Read the model definition and answer for the solid it produces. Units are mm, in the model's axes. A direction names the side the tool comes from. Round coordinates to 2 decimals unless told otherwise and drop trailing zeros. Write each loop counter-clockwise with the first axis right and the second up, starting at its lowest first coordinate (ties: lowest second). Pieces come first, ordered by that corner, then holes. Notation, with made-up numbers: (89, -33.75) -> (120, -33.75) arc R20 cw to (120, -23.75) -> close; hole circle Ø8 at (88, 85). An arc over 180 degrees is marked (long way). Return JSON: item names as keys, results as strings. Group by question number.
(1) The mould has two halves that part along Y. Classify faces 1 (the flat face through (0, -3.175, -7)), 2 (the cylindrical face through (-0.01, -5.62, 6.54)), 3 (the flat face through (-5, 1, -11.112)): released by +Y, released by -Y, zero draft, split by the parting line, or undercut.
(2) A cutting plane is placed at C-C on y = 0. Give the vertices of the cut face in (x, z) (1 decimal).
(3) A cutting plane is placed at A-A on z = 8.75. Give the vertices of the cut face in (x, y), then the cut area to 3 significant figures.
(4) A cutting plane is placed at D-D on z = -4.5. Give the vertices of the cut face in (x, y) (3 decimals), then the cut area to 3 significant figures.
(5) For faces 4 (the flat face through (-3.175, 0, -7)), 5 (the flat face through (2, 6, 11.112)), 6 (the cylindrical face through (-4.87, -2.8, 6.54)), determine the directions among +Z, -Z, +X, -X, +Y, -Y from which every point of the face is accessible in a straight line to the end or side of a thin tool.
(6) Straight lines are drawn through the part: line 1 (Y direction, x = 0, z = -1.05); line 2 (X direction, y = 0.25, z = -6.75) (3 decimals); line 3 (Z direction, x = -4.5, y = 3). For each, find the intervals that lie inside material, in ascending order.
(7) Given pin 1 (1.5 mm diameter, centred on y = 5.5, z = 8, fed in from +X); pin 2 (0.9 mm diameter, centred on x = 3.5, y = -1, fed in from +Z); pin 3 (7 mm diameter, centred on x = 0, y = 0, fed in from -Z), each flat-ended and moving along its own axis, determine where each tip first touches the part or whether it passes through.
```python
from build123d import *

# Parameters (mm, degrees)
SKETCH4_W          = 22.225
SKETCH4_H          = 7.3421875
CUT_EXTRUDE1_DEPTH = 9.128125
CUT_EXTRUDE3_START = -4.7625
SKETCH7_R          = 4
CUT_EXTRUDE3_DEPTH = 4.7625
SKETCH9_W          = 6.35
SKETCH9_H          = 6.35
CUT_EXTRUDE5_DEPTH = 8.334375
FILLET1_R          = 0.3175


with BuildPart() as part:
    # Sketch4 → Revolve1 (revolve)
    with BuildSketch(Plane(origin=(0, 0, 0), x_dir=(0, 0, -1), z_dir=(1, 0, 0)), mode=Mode.PRIVATE) as revolve1_sk:
        with Locations((0, 3.67109375)):
            Rectangle(SKETCH4_W, SKETCH4_H)
    revolve(revolve1_sk.sketch.rotate(Axis((0, 0, 11.1125), (0, 0, -1)), 90), axis=Axis((0, 0, 11.1125), (0, 0, -1)))

    # Sketch5 → Cut-Extrude1 (cut)
    with BuildSketch(Plane.XY.offset(11.1125)):
        with BuildLine():
            Line((-5, 2.309401077), (-5, -2.309401077))
            ThreePointArc((-5, -2.309401077), (-4.866025404, -2.809401077), (-4.5, -3.175426481))
            Line((-4.5, -3.175426481), (-0.5, -5.484827557))
            ThreePointArc((-0.5, -5.484827557), (0, -5.618802154), (0.5, -5.484827557))
            Line((0.5, -5.484827557), (4.5, -3.175426481))
            ThreePointArc((4.5, -3.175426481), (4.866025404, -2.809401077), (5, -2.309401077))
            Line((5, -2.309401077), (5, 2.309401077))
            ThreePointArc((5, 2.309401077), (4.866025404, 2.809401077), (4.5, 3.175426481))
            Line((4.5, 3.175426481), (0.5, 5.484827557))
            ThreePointArc((0.5, 5.484827557), (0, 5.618802154), (-0.5, 5.484827557))
            Line((-0.5, 5.484827557), (-4.5, 3.175426481))
            ThreePointArc((-4.5, 3.175426481), (-4.866025404, 2.809401077), (-5, 2.309401077))
        make_face()
    extrude(amount=-CUT_EXTRUDE1_DEPTH, mode=Mode.SUBTRACT)

    # Sketch7 → Cut-Extrude3 (cut)
    with BuildSketch(Plane.XY.offset(1.984375).offset(CUT_EXTRUDE3_START)):
        Circle(SKETCH7_R)
    extrude(amount=CUT_EXTRUDE3_DEPTH, mode=Mode.SUBTRACT)

    # Sketch9 → Cut-Extrude5 (cut)
    with BuildSketch(Plane(origin=(0, 0, -11.1125), x_dir=(-1, 0, 0), z_dir=(0, 0, -1))):
        Rectangle(SKETCH9_W, SKETCH9_H)
    extrude(amount=-CUT_EXTRUDE5_DEPTH, mode=Mode.SUBTRACT)

    # Cut-Extrude6 cone 1 section (through the dimple's axis) → Cut-Extrude6 (revolve, cut)
    with BuildSketch(Plane(origin=(0, 0, -11.1125), x_dir=(0, 1, 0), z_dir=(1, 0, 0))):
        Polygon((0, 0), (4.744128061, 0), (0, 2.739023613), align=None)
    revolve(axis=Axis((0, 0, -11.1125), (0, 0, 1)), mode=Mode.SUBTRACT)

    # Fillet1
    fillet1_edges = [part.edges().sort_by_distance(p)[0] for p in [
        (-7.3421875, 0, -11.1125),
        (-7.3421875, 0, 11.1125),
    ]]
    fillet(fillet1_edges, radius=FILLET1_R)

    # Cut-Extrude9 cone 1 section (through the dimple's axis) → Cut-Extrude9 (revolve, cut)
    with BuildSketch(Plane(origin=(0, 0, 11.1125), x_dir=(0, -1, 0), z_dir=(1, 0, 0))):
        Polygon((0, 0), (5.872802154, 0), (0, 3.390663904), align=None)
    revolve(axis=Axis((0, 0, 11.1125), (0, 0, -1)), mode=Mode.SUBTRACT)


solid = part.part
```
Checks:
{
 "1": {"face 1": "undercut", "face 2": "undercut", "face 3": "zero draft"},
 "2": {"outline": "(-7.3, -10.8) arc R0.3 ccw to (-7, -11.1) -> (-4.7, -11.1) -> (-3.2, -10.2) -> (-3.2, -2.8) -> (-4, -2.8) -> (-4, 2) -> (-5, 2) -> (-5, 10.6) -> (-5.9, 11.1) -> (-7, 11.1) arc R0.3 ccw to (-7.3, 10.8) -> close; (3.2, -10.2) -> (4.7, -11.1) -> (7, -11.1) arc R0.3 ccw to (7.3, -10.8) -> (7.3, 10.8) arc R0.3 ccw to (7, 11.1) -> (5.9, 11.1) -> (5, 10.6) -> (5, 2) -> (4, 2) -> (4, -2.8) -> (3.2, -2.8) -> close"},
 "3": {"outline": "circle Ø14.68 at (0, 0); hole (-5, -2.31) arc R1 ccw to (-4.5, -3.18) -> (-0.5, -5.48) arc R1 ccw to (0.5, -5.48) -> (4.5, -3.18) arc R1 ccw to (5, -2.31) -> (5, 2.31) arc R1 ccw to (4.5, 3.18) -> (0.5, 5.48) arc R1 ccw to (-0.5, 5.48) -> (-4.5, 3.18) arc R1 ccw to (-5, 2.31) -> close", "area": "83.1 mm^2"},
 "4": {"outline": "circle Ø14.684 at (0, 0); hole (-3.175, -3.175) -> (3.175, -3.175) -> (3.175, 3.175) -> (-3.175, 3.175) -> close", "area": "129 mm^2"},
 "5": {"face 4": "-Z", "face 5": "+Z, +X, -X, +Y, -Y", "face 6": "+Z"},
 "6": {"line 1": "y = -7.34 to -4, 4 to 7.34", "line 2": "x = -7.338 to -3.175, 3.175 to 7.338", "line 3": "z = -11.11 to 1.98"},
 "7": {"pin 1": "stops at x = 5.6", "pin 2": "stops at z = 1.98", "pin 3": "stops at z = -10.39"}
}
